Part model, mm, in its own coordinate system. A direction names the side the tool comes from. Round coordinates to 2 decimals unless told otherwise and drop trailing zeros. Order: outer loops, then holes, each group sorted by start corner. A loop starts at its lowest first (then second) coordinate and runs counter-clockwise, first axis right, second up. Notation, with made-up numbers: (53.25, 48.5) - (85.25, 48.5) arc R9 cw to (85.25, 57.5) - close; hole circle Ø10 at (68.25, 84). An arc over 180 degrees is marked (long way). Answer as a JSON object with one key per item and string values.
```python
from build123d import *

# Parameters (mm, degrees)
BOSS_EXTRUDE1_DEPTH = 1066.8
SKETCH2_R           = 2.45745
CUT_EXTRUDE1_DEPTH  = 889


with BuildPart() as part:
    # Sketch1 → Boss-Extrude1 (new body)
    with BuildSketch(Plane(origin=(0, 0, 0), x_dir=(0, 0, -1), z_dir=(1, 0, 0))):
        Polygon((0, 0), (0, 44.45), (3.175, 44.45), (3.175, 3.175), (44.45, 3.175), (44.45, 0), align=None)
    extrude(amount=BOSS_EXTRUDE1_DEPTH)

    # Sketch2 → Cut-Extrude1 (cut)
    with BuildSketch(Plane(origin=(0, 3.175, 0), x_dir=(1, 0, 0), z_dir=(0, 1, 0))):
        with Locations(Location((120.65, 22.225, 0), (0, 0, 270))):
            Circle(SKETCH2_R)
        with Locations(Location((395.81582, 22.225, 0), (0, 0, 270))):
            Circle(SKETCH2_R)
        with Locations(Location((670.98418, 22.225, 0), (0, 0, 270))):
            Circle(SKETCH2_R)
        with Locations(Location((946.15, 22.225, 0), (0, 0, 270))):
            Circle(SKETCH2_R)
    extrude(amount=-CUT_EXTRUDE1_DEPTH, mode=Mode.SUBTRACT)


solid = part.part
```
Item 1: Cut at A-A (x = 588.5). Write the cut outline in (y, z) (3 decimals), plus the area to 3 significant figures.
Taken from the geometry:
{"outline": "(0, -44.45) - (3.175, -44.45) - (3.175, -3.175) - (44.45, -3.175) - (44.45, 0) - (0, 0) - close", "area": "272 mm2"}
Item 2: Tool access for faces 1 (the flat face through (526, 22, 0)), 2 (the flat face through (526, 3.175, -24)): list every direction of +Z, -Z, +X, -X, +Y, -Y with a clear straight run to the whole face (end or side of a thin tool).
Taken from the geometry:
{"face 1": "+Z, +X, -X, +Y, -Y", "face 2": "-Z, +X, -X, +Y"}
Item 3: Probe L1, parallel to Z at x = 120, y = 1; L2, parallel to Z at x = 581, y = 39 (3 decimals); L3, parallel to Y at x = 53, z = -30.5 (3 decimals). List the from-to ranges inside material, lowest first. Write a range as from..to.
Taken from the geometry:
{"L1": "-44.45..-24.59, -19.86..0", "L2": "-3.175..0", "L3": "0..3.175"}
Item 4: Cut at B-B (y = 20). Write the cut outline in (x, z) (3 decimals), plus the area to 3 significant figures.
Taken from the geometry:
{"outline": "(0, -3.175) - (1066.8, -3.175) - (1066.8, 0) - (0, 0) - close", "area": "3,390 mm2"}
Item 5: Drop flat-ended pins along their axis: P1, Ø4.5, axis at x = 395.82, z = -22.22, coming from the -Y side; P2, Ø12.5, axis at x = 356, y = 25, coming from the -Z side (3 decimals); P3, Ø4, axis at x = 218, y = 39, coming from the +Z side; P4, Ø12.5, axis at x = 268, z = -24, coming from the +Y side (3 decimals). Give the stop position or say it passes through.
Taken from the geometry:
{"P1": "through", "P2": "z = -3.175", "P3": "z = 0", "P4": "y = 3.175"}
